Design review of the part built by this model. Coordinates are the model's own, in mm. A direction names the side the tool comes from. Give positions to 0.01 mm unless a question says otherwise; leave off trailing zeros. Loops run counter-clockwise (first coordinate to the right, second up) from the corner with the lowest first, then second, coordinate; pieces in that order, holes last. Notation, with made-up numbers: (-35, -11) - (9, -11) arc R12 cw to (9, -7) - close; hole circle Ø10 at (77, -33). An arc over 180 degrees is marked (long way). Put each result on its own line as item: value. Start each with the question number.
```python
from build123d import *

# Parameters (mm, degrees)
BOSS_EXTRUDE1_DEPTH = 3.175
CUT_EXTRUDE1_DEPTH  = 7.35
CUT_EXTRUDE2_DEPTH  = 7.62


with BuildPart() as part:
    # Sketch1 → Boss-Extrude1 (new body, symmetric)
    with BuildSketch(Plane.XY):
        Polygon((76.2, 37.697541537), (76.2, 56.747541537), (79.375, 56.747541537), (79.375, 37.697541537), (92.075, 37.697541537), (92.075, 46.587541537), (95.25, 46.587541537), (95.25, 37.697541537), (136.525, 37.697541537), (136.525, 46.587541537), (139.7, 46.587541537), (139.7, 37.697541537), (152.4, 37.697541537), (152.4, 69.447541537), (0, 69.447541537), (-0.423998633, 69.491926731), (-3.587863461, 69.757603883), (-946.051908629, 122.953392794), (-946.583462345, 116.623288424), (-943.412318182, 116.444298555), (-943.91275138, 110.48479854), (-6.775989292, 31.791225946), (-5.713280681, 44.446685258), (-2.549415853, 44.181008106), (-3.612124464, 31.525548794), (-1.492292584, 31.347541537), (0, 31.347541537), (0, 44.047541537), (3.175, 44.047541537), (3.175, 31.347541537), (15.875, 31.347541537), (15.875, 36.427541537), (19.05, 36.427541537), (19.05, 31.347541537), (25.4, 31.347541537), (69.85, 37.697541537), align=None)
    extrude(amount=BOSS_EXTRUDE1_DEPTH, both=True)

    # Sketch2 → Cut-Extrude1 (cut, through all)
    with BuildSketch(Plane.XY.offset(3.175)):
        Polygon((-76.254460917, 37.625496217), (-75.245037036, 49.646404609), (-78.411328309, 49.883186), (-79.418325745, 37.891173369), align=None)
        Polygon((-155.224527027, 44.256797945), (-154.27566721, 55.556468134), (-157.441958483, 55.793249525), (-158.388391855, 44.522475098), align=None)
        Polygon((-234.194593137, 50.888099674), (-233.306297384, 61.466531659), (-236.472588657, 61.70331305), (-237.358457965, 51.153776826), align=None)
        Polygon((-313.164659247, 57.519401402), (-312.336927558, 67.376595183), (-315.503218831, 67.613376574), (-316.328524075, 57.785078555), align=None)
        Polygon((-392.134725356, 64.15070313), (-391.367557732, 73.286658708), (-394.533849005, 73.523440099), (-395.298590185, 64.416380283), align=None)
        Polygon((-471.104791466, 70.782004859), (-470.398187906, 79.196722233), (-473.564479179, 79.433503624), (-474.268656294, 71.047682011), align=None)
        Polygon((-550.074857576, 77.413306587), (-549.42881808, 85.106785757), (-552.595109353, 85.343567149), (-553.238722404, 77.67898374), align=None)
        Polygon((-629.044923686, 84.044608316), (-628.459448254, 91.016849282), (-631.625739527, 91.253630673), (-632.208788514, 84.310285468), align=None)
        Polygon((-708.014989796, 90.675910044), (-707.490078428, 96.926912807), (-710.656369701, 97.163694198), (-711.178854624, 90.941587197), align=None)
        Polygon((-786.985055905, 97.307211772), (-786.520708602, 102.836976331), (-789.686999875, 103.073757723), (-790.148920734, 97.572888925), align=None)
        Polygon((-865.955122015, 103.938513501), (-865.551338776, 108.747039856), (-868.717630049, 108.983821247), (-869.118986843, 104.204190653), align=None)
    extrude(amount=-CUT_EXTRUDE1_DEPTH, mode=Mode.SUBTRACT)

    # Sketch3 → Cut-Extrude2 (cut)
    with BuildSketch(Plane.XY.offset(3.175)):
        Polygon((-354.231624716, 60.967890842), (-362.126685184, 71.979397876), (-347.872352174, 77.449083798), (-357.599036746, 89.739165772), (-993.791218606, 254.183288708), (-993.791218606, 28.735079887), align=None)
    extrude(amount=-CUT_EXTRUDE2_DEPTH, mode=Mode.SUBTRACT)


solid = part.part
```
Item 1: Consider section A-A (x = 106). State the section outline as (y, z) points (3 decimals), plus the area to 3 significant figures.
Item 2: Consider section B-B (x = -120.5). State the section outline as (y, z) points (3 decimals).
Item 3: Machinability: for faces 1 (the flat face through (-352.67, 83.51, 0.04)), 2 (the flat face through (-108, 61, 3.175)), which of the approach directions +Z, -Z, +X, -X, +Y, -Y give a long, thin tool a straight path to every point of the face, cutting with its end or side? Answer none if there is none.
Item 4: For P1, Ø3, axis at y = 69.5, z = 1.5, coming from the +X side; P2, Ø1.6, axis at x = 18, z = -1, coming from the -Y side; P3, Ø1, axis at x = 78.5, z = 0, coming from the -Y side; P4, Ø3, axis at x = -85.5, z = -2, coming from the -Y side, all flat-tipped, find the tip position at first contact; note any pin that passes through.
Item 5: For L1, parallel to X at y = 51, z = 2.5 (3 decimals); L2, parallel to Y at x = 116, z = 2.5; L3, parallel to Y at x = 17.5, z = -1.5, list the stretches that pass through material, from the lowest coordinate up. Write a range as from..to.
Geometry says:
1. outline: (37.698, -3.175) - (69.448, -3.175) - (69.448, 3.175) - (37.698, 3.175) - close
1. area: 202 mm2
2. outline: (41.341, -3.175) - (76.357, -3.175) - (76.357, 3.175) - (41.341, 3.175) - close
3. face 1: +Z, -Z, -X
3. face 2: +Z, +X, -X, +Y, -Y
4. P1: stops at x = 152.4
4. P2: stops at y = 36.43
4. P3: stops at y = 56.75
4. P4: stops at y = 38.28
5. L1: x = -234.185..-157.844, -154.658..76.2, 79.375..152.4
5. L2: y = 37.7..69.45
5. L3: y = 36.43..69.45
